Can you work these out from the model? Positions are in its coordinate system, mm. A direction names the side the tool comes from. Coordinates: 2 decimals unless noted, no trailing zeros. Order: outer loops, then holes, each group sorted by start corner. A loop starts at its lowest first (then second) coordinate and runs counter-clockwise, first axis right, second up. Notation, with made-up numbers: (-16.75, 66) -> (28.25, 66) arc R14 cw to (28.25, 79) -> close; hole circle Ø4 at (-35.5, -23.5). An arc over 180 degrees is marked (long way). Answer in a Markdown table with one row per item. Add a question column.
1. Will these pins go through, and if not, where does the flat tip stop? pin 1 (25 mm diameter, centred on y = -75.5, z = 34, fed in from -X); pin 2 (8 mm diameter, centred on x = -274, y = -72, fed in from -Z); pin 3 (15 mm diameter, centred on y = -17, z = 272.5, fed in from +X).
2. We'd pull the mould along Y, two halves only. Please class faces 5 (the face through (14.43, -270.42, 514.026)), 6 (the face through (559, 3, 250)): pulls with the +Y half, pulls with the -Y half, needs draft (parallel to the pull), parting line crosses it, or undercut.
3. If I drill on line 1 along Y through (x, z) = (-353, 374); line 2 along Z through (x, y) = (244.5, 57.5); line 3 along Z through (x, y) = (-279, -79), over which ranges is the centre line in solid material (lowest first)? Write a range as [from, to].
4. Imagine slicing it at D-D on y = 179. Write out the boundary of the cut face in (x, z).
5. Imagine slicing it at B-B on z = 419.5. Write out the boundary of the cut face in (x, y).
6. Imagine slicing it at A-A on y = 0. Write out the boundary of the cut face in (x, z), plus the area to 3 significant figures.
7. On a 3-axis mill with a long thin cutter (end or side, diameter ignored), from which of +Z, -Z, +X, -X, +Y, -Y can I reach the whole of each face in a straight line? I mean faces 1 (the face through (-4, 110, 300)), 2 (the face through (275, -3, 275)), 3 (the face through (-566, 3, 250)), 4 (the face through (-196.124, 2.199, 226.05)). Say none if no direction works.
8. Imagine slicing it at C-C on x = 61.5. Write out the boundary of the cut face in (y, z), plus the area to 3 significant figures.
from build123d import *

# Parameters (mm, degrees)
F0_W      = 1700
F0_H      = 480
F1_DEPTH  = 250
F2_W      = 1700
F2_H      = 60
F3_DEPTH  = 250
F5_DEPTH  = 60
F7_DEPTH  = 60
F8_W      = 550
F8_H      = 480
F9_DEPTH  = 50
F11_DEPTH = 300.001
F12_W     = 700
F12_H     = 300
F13_DEPTH = 600.001
F14_W     = 403.557981
F14_H     = 200
F15_DEPTH = 600.001
F16_R     = 50
F17_W     = 396.442019
F17_H     = 200
F18_DEPTH = 600.001
F19_R     = 50


with BuildPart() as f1:
    # F0 (on Top) → F1 (new body)
    with BuildSketch(Plane.XY):
        with Locations((1.77899, 0)):
            Rectangle(F0_W, F0_H)
    extrude(amount=F1_DEPTH)

    # F2 (on face) → F3 (join)
    with BuildSketch(Plane.XY.offset(250)):
        with Locations((1.77899, -270)):
            Rectangle(F2_W, F2_H)
        with Locations((1.77899, 270)):
            Rectangle(F2_W, F2_H)
    extrude(amount=-F3_DEPTH)

    # F4 (on face) → F5 (join)
    with BuildSketch(Plane.XZ.offset(300)):
        with BuildLine():
            Line((-848.22101, 250), (851.77899, 250))
            ThreePointArc((851.77899, 250), (1.77899, 514.079291), (-848.22101, 250))
        make_face()
    extrude(amount=-F5_DEPTH)

    # F6 (on face) → F7 (join)
    with BuildSketch(Plane(origin=(0, 300, 0), x_dir=(-1, 0, 0), z_dir=(0, 1, 0))):
        with BuildLine():
            Line((-851.77899, 250), (848.22101, 250))
            ThreePointArc((848.22101, 250), (-1.77899, 514.079291), (-851.77899, 250))
        make_face()
    extrude(amount=-F7_DEPTH)

    # F8 (on face) → F9 (join)
    with BuildSketch(Plane.XY.offset(250)):
        Rectangle(F8_W, F8_H)
    extrude(amount=F9_DEPTH)

    # F10 (on face) → F11 (cut, through all)
    with BuildSketch(Plane.XY.offset(300)):
        with BuildLine():
            Line((-96.148637, -100), (103.851363, -100))
            ThreePointArc((103.851363, -100), (203.851363, 0), (103.851363, 100))
            Line((103.851363, 100), (-96.148637, 100))
            ThreePointArc((-96.148637, 100), (-196.148637, 0), (-96.148637, -100))
        make_face()
    extrude(amount=-F11_DEPTH, mode=Mode.SUBTRACT)

    # F12 (on face) → F13 (cut, through all)
    with BuildSketch(Plane.XZ.offset(300)):
        Rectangle(F12_W, F12_H)
    extrude(amount=-F13_DEPTH, mode=Mode.SUBTRACT)

    # F14 (on face) → F15 (cut, through all)
    with BuildSketch(Plane.XZ.offset(300)):
        with Locations((-848.22101, 0)):
            Rectangle(F14_W, F14_H)
    extrude(amount=-F15_DEPTH, mode=Mode.SUBTRACT)

    # F16
    f16_edges = [f1.edges().sort_by_distance(p)[0] for p in [
        (-646.442019, 0, 100),
    ]]
    fillet(f16_edges, radius=F16_R)

    # F17 (on face) → F18 (cut, through all)
    with BuildSketch(Plane.XZ.offset(300)):
        with Locations((851.77899, 0)):
            Rectangle(F17_W, F17_H)
    extrude(amount=-F18_DEPTH, mode=Mode.SUBTRACT)

    # F19
    f19_edges = [f1.edges().sort_by_distance(p)[0] for p in [
        (653.557981, 0, 100),
    ]]
    fillet(f19_edges, radius=F19_R)


solid = f1.part
Answers follow:
| question | item | result |
|---|---|---|
| 1 | pin 1 | stops at x = -646.44 |
| 1 | pin 2 | stops at z = 150 |
| 1 | pin 3 | stops at x = 275 |
| 2 | face 5 | needs draft |
| 2 | face 6 | undercut |
| 3 | line 1 | y = [-300, -240], [240, 300] |
| 3 | line 2 | z = [150, 300] |
| 3 | line 3 | z = [150, 250] |
| 4 | outline | (-848.22, 100) -> (-696.44, 100) arc R50 cw to (-646.44, 50) -> (-646.44, 0) -> (-350, 0) -> (-350, 150) -> (350, 150) -> (350, 0) -> (653.56, 0) -> (653.56, 50) arc R50 cw to (703.56, 100) -> (851.78, 100) -> (851.78, 250) -> (275, 250) -> (275, 300) -> (-275, 300) -> (-275, 250) -> (-848.22, 250) -> close |
| 5 | outline | (-522.43, -300) -> (525.99, -300) -> (525.99, -240) -> (-522.43, -240) -> close; (-522.43, 240) -> (525.99, 240) -> (525.99, 300) -> (-522.43, 300) -> close |
| 6 | outline | (-848.22, 100) -> (-696.44, 100) arc R50 cw to (-646.44, 50) -> (-646.44, 0) -> (-350, 0) -> (-350, 150) -> (-196.15, 150) -> (-196.15, 300) -> (-275, 300) -> (-275, 250) -> (-848.22, 250) -> close; (203.85, 150) -> (350, 150) -> (350, 0) -> (653.56, 0) -> (653.56, 50) arc R50 cw to (703.56, 100) -> (851.78, 100) -> (851.78, 250) -> (275, 250) -> (275, 300) -> (203.85, 300) -> close |
| 6 | area | 249,000 mm² |
| 7 | face 1 | +Z, +X, -X |
| 7 | face 2 | +Z, +X |
| 7 | face 3 | +Z, -X |
| 7 | face 4 | +Z, -Z |
| 8 | outline | (-300, 150) -> (-100, 150) -> (-100, 300) -> (-240, 300) -> (-240, 512.89) -> (-300, 512.89) -> close; (100, 150) -> (300, 150) -> (300, 512.89) -> (240, 512.89) -> (240, 300) -> (100, 300) -> close |
| 8 | area | 85,500 mm² |
